Part model, mm, in its own coordinate system. A direction names the side the tool comes from. Round coordinates to 2 decimals unless told otherwise and drop trailing zeros. Write each loop counter-clockwise with the first axis right and the second up, starting at its lowest first coordinate (ties: lowest second). Pieces come first, ordered by that corner, then holes. Notation, with made-up numbers: (-4, 73.25) -> (20, 73.25) arc R16 cw to (20, 94.25) -> close; hole circle Ø7 at (79.5, 25.5). An arc over 180 degrees is marked (long way). Return JSON: item names as keys, results as strings. Group by question number.
```python
from build123d import *

# Parameters (mm, degrees)
EXTRUDE_3_DEPTH = 3
SKETCH_4_R      = 15
EXTRUDE_4_DEPTH = 1


with BuildPart() as part:
    # 草图3 → 凸台-拉伸3 (new body)
    with BuildSketch(Plane(origin=(0, 0, 0), x_dir=(1, 0, 0), z_dir=(0, 1, 0))):
        Polygon((170, 190), (170, 170), (190, 170), (190, -170), (170, -170), (170, -190), (-170, -190), (-170, -170), (-190, -170), (-190, 170), (-170, 170), (-170, 190), align=None)
    extrude(amount=EXTRUDE_3_DEPTH)

    # 草图4 → 凸台-拉伸4 (add)
    with BuildSketch(Plane.XZ):
        with Locations(Location((0, 0, 0), (0, 0, 270))):
            Circle(SKETCH_4_R)
    extrude(amount=EXTRUDE_4_DEPTH)


solid = part.part
```
Item 1: Wall check: L1, parallel to Y at x = -165.5, z = -68.5; L2, parallel to Z at x = -173.5, y = 1.35. Give the ranges that are in metal, low to high.
Item 2: Cut at A-A (z = 0). Write the cut outline in (x, y).
Item 3: Cut at B-B (x = 0). Write the cut outline in (y, z), then the cut area to 3 significant figures.
Item 4: Flat gauge pins, fed straight in: P1, Ø0.9, axis at x = -181.5, y = 1, coming from the +Z side; P2, Ø0.9, axis at x = 178.5, y = 1.5, coming from the -Z side; P3, Ø1, axis at x = -17, z = -94.5, coming from the -Y side. Where does each tip first touch, or does it go through?
Item 5: Cut at D-D (x = -119). Write the cut outline in (y, z), then the cut area to 3 significant figures.
Item 6: Which spindle directions (+Z, -Z, +X, -X, +Y, -Y) get a long thin tool onto all of the face, cutting with end or side? Do faces 1 (the face through (0.66, -0.493, 14.985)), 2 (the face through (3, 3, -3)). Say none if no direction does.
Item 7: Cut at C-C (z = -60). Write the cut outline in (x, y).
Checks:
{
 "1": {"L1": "y = 0 to 3", "L2": "z = -170 to 170"},
 "2": {"outline": "(-190, 0) -> (-15, 0) -> (-15, -1) -> (15, -1) -> (15, 0) -> (190, 0) -> (190, 3) -> (-190, 3) -> close"},
 "3": {"outline": "(-1, -15) -> (0, -15) -> (0, -190) -> (3, -190) -> (3, 190) -> (0, 190) -> (0, 15) -> (-1, 15) -> close", "area": "1,170 mm2"},
 "4": {"P1": "stops at z = 170", "P2": "stops at z = -170", "P3": "stops at y = 0"},
 "5": {"outline": "(0, -190) -> (3, -190) -> (3, 190) -> (0, 190) -> close", "area": "1,140 mm2"},
 "6": {"face 1": "-Y", "face 2": "+Z, -Z, +X, -X, +Y"},
 "7": {"outline": "(-190, 0) -> (190, 0) -> (190, 3) -> (-190, 3) -> close"}
}
